CAD build for the part. Positions are in the model's coordinates, mm. A direction names the side the tool comes from. Round coordinates to 2 decimals unless told otherwise and drop trailing zeros. Loops run counter-clockwise (first coordinate to the right, second up) from the corner with the lowest first, then second, coordinate; pieces in that order, holes last. Notation, with made-up numbers: M 2.25,86.5 L 20.25,86.5 A22 ccw 20.25,97.5 Z; hole C 43.25,-13 d6. An arc over 180 degrees is marked long. Put each result on its own line as item: value. Start each with the question number.
Autodesk Inventor part; units mm, degrees
ref_plane "YZ Plane" through (0, 0, 0) normal (1, 0, 0) x (0, 1, 0)
ref_plane "XZ Plane" through (0, 0, 0) normal (0, 1, 0) x (-1, 0, 0)
ref_plane "XY Plane" through (0, 0, 0) normal (0, 0, 1) x (1, 0, 0)
sketch "스케치2" plane through (0, 0, 0) normal (0, 1, 0) x (-1, 0, 0)
  line L0 (0, -70.4) -> (-60.9682, -35.2)
  line L1 (-60.9682, -35.2) -> (-60.9682, 35.2)
  line L2 (-60.9682, 35.2) -> (0, 70.4)
  line L3 (0, 70.4) -> (60.9682, 35.2)
  line L4 (60.9682, 35.2) -> (60.9682, -35.2)
  line L5 (60.9682, -35.2) -> (0, -70.4)
  line L6 (60.9682, -35.2) -> (-60.9682, -35.2)
  line L7 (-60.9682, -35.2) -> (-60.9682, 35.2)
  line L8 (-60.9682, 35.2) -> (60.9682, 35.2)
  line L9 (60.9682, 35.2) -> (60.9682, -35.2)
  line L10 (60.9682, -35.2) -> (-60.9682, 35.2) construction
  line L11 (-60.9682, -35.2) -> (60.9682, 35.2) construction
  line L12 (0, 76.1735) -> (-65.9682, 38.0868)
  line L13 (-65.9682, 38.0868) -> (-65.9682, -38.0868)
  line L14 (-65.9682, -38.0868) -> (0, -76.1735)
  line L15 (0, -76.1735) -> (65.9682, -38.0868)
  line L16 (65.9682, -38.0868) -> (65.9682, 38.0868)
  line L17 (65.9682, 38.0868) -> (0, 76.1735)
  line L18 (49.325, -35.2) -> (-49.325, -35.2)
  line L19 (-49.325, -35.2) -> (-49.325, 35.2)
  line L20 (-49.325, 35.2) -> (49.325, 35.2)
  line L21 (49.325, 35.2) -> (49.325, -35.2)
  line L22 (49.325, -35.2) -> (-49.325, 35.2) construction
  line L23 (-49.325, -35.2) -> (49.325, 35.2) construction
  line L24 (49.325, 35.2) -> (65.9682, 35.2)
  line L25 (65.9682, 35.2) -> (65.9682, 29.2)
  line L26 (65.9682, 29.2) -> (49.325, 29.2)
  line L27 (49.325, 29.2) -> (49.325, 35.2)
  line L28 (49.325, -35.2) -> (65.9682, -35.2)
  line L29 (65.9682, -35.2) -> (65.9682, -29.2)
  line L30 (65.9682, -29.2) -> (49.325, -29.2)
  line L31 (49.325, -29.2) -> (49.325, -35.2)
  line L32 (5.675, -35.2) -> (5.675, -72.897)
  line L33 (-49.325, -25.2) -> (-65.9682, -25.2)
  line L34 (-65.9682, -25.2) -> (-65.9682, -5.2)
  line L35 (-65.9682, -5.2) -> (-49.325, -5.2)
  line L36 (-49.325, -5.2) -> (-49.325, -25.2)
  line L37 (-39.325, -35.2) -> (-39.325, -53.4692)
  point P0 (0, 0)
  point P1 (0, 0)
  dimension "d2" = 70.4
  dimension "d3" = 70.4
  dimension "d4" = 5
  dimension "d5" = 98.65
  dimension "d6" = 6
  dimension "d7" = 6
  dimension "d9" = 10
  dimension "d10" = 30
  dimension "d15" = 10
  dimension "d16" = 55
extrude "돌출1" add sketch "스케치2" along normal blind 32 contours L37 L14 L13 L33 L1 L0 | L0 L6 L37 | L32 L6 L5 | L5 L28 L16 L15 L32 | L1 L33 L19 L6 | L6 L21 L30 L4 | L4 L30 L16 L28 | L35 L13 L12 L17 L16 L24 L3 L2 L1 | L1 L8 L19 L35 | L26 L21 L8 L4 | L4 L24 L16 L26 | L2 L3 L8
sketch "스케치3" plane through (0, 0, 0) normal (0, 1, 0) x (-1, 0, 0)
  line L0 (0, 76.1735) -> (-65.9682, 38.0868) construction
  line L1 (0, 76.1735) -> (65.9682, 38.0868)
  line L2 (65.9682, 38.0868) -> (65.9682, -38.0868)
  line L3 (65.9682, -38.0868) -> (0, -76.1735)
  line L4 (0, -76.1735) -> (-65.9682, -38.0868)
  line L5 (-65.9682, -38.0868) -> (-65.9682, 38.0868)
  line L6 (-65.9682, 38.0868) -> (0, 76.1735)
  point P0 (0, 0)
  point P1 (0, 0)
extrude "돌출2" add sketch "스케치3" against normal blind 5
sketch "스케치4" plane through (0, 32, 0) normal (0, 1, 0) x (1, 0, 0)
  circle A0 centre (0, -55) radius 2.5
  circle A1 centre (-25, 45) radius 2.5
  circle A2 centre (57, 35) radius 2.5
  point P0 (0, 0)
  dimension "d17" = 5
  dimension "d18" = 55
  dimension "d19" = 5
  dimension "d20" = 45
  dimension "d21" = 25
  dimension "d22" = 5
  dimension "d23" = 57
  dimension "d24" = 35
extrude "돌출3" cut sketch "스케치4" against normal blind 5
chamfer "모따기1" distance 1 angle 45 10 edges at (-2.5, 32, 55) (-27.5, 32, -45) (54.5, 32, -35) (-27.5, 32, -35.2) (-49.325, 32, -32.2) (-49.325, 32, 32.2) (0, 32, 35.2) (44.325, 32, -35.2) (49.325, 32, -30.2) (49.325, 32, 15)
equation "\"d3\" = d2"
properties part number "pi_case_bottom"
(1) Cut at B-B on y = 24. List the corners of the cut face in (x, z) (1 decimal), and give its area (3 significant figures).
(2) Cut at D-D on z = -59. List the corners of the cut face in (x, y) (3 decimals).
(3) Cut at C-C on x = -44.5. List the corners of the cut face in (y, z), and give its area (3 significant figures).
(4) Flat gauge pins, fed straight in: pin 1 Ø12 at (x, y) = (33, 13) entering from +Z; pin 2 Ø5.5 at (x, z) = (58, -35.5) entering from +Y; pin 3 Ø9.5 at (x, y) = (-16, 17.5) entering from -Z; pin 4 Ø4 at (x, y) = (-34.5, 26) entering from +Z. Where does each tip first touch, or does it go through?
(5) Cut at A-A on z = 2. List the corners of the cut face in (x, y) (3 decimals).
(6) Drill centre lines: line 1 along X through (y, z) = (29, -35) (3 decimals); line 2 along Z through (x, y) = (0, 29.05); line 3 along Z through (x, y) = (57, 27.85). Where is each one in solid material? Low to high.
(7) Tool access for faces 1 (the flat face through (-32.52, 13.76, 57.4)), 2 (the flat face through (1, 0, -7)), 3 (the flat face through (10, 32, 42)), 4 (the flat face through (58, 16, -5.2)), 5 (the flat face through (-58, 16, 29.2)): list every direction of +Z, -Z, +X, -X, +Y, -Y with a clear straight run to the whole face (end or side of a thin tool).
(8) Mould opens along Z. For faces 6 (the flat face through (49.325, 15, -30)), 7 (the flat face through (39.325, 16, -44)), 8 (the flat face through (-33.45, 13.76, -56.86)) say: +Z half, -Z half, draft (parallel to the pull), parting line (faces both ways), or undercut.
Taken from the geometry:
1. outline: M -66,-38.1 L -5.7,-72.9 L -5.7,-35.2 L -49.3,-35.2 L -49.3,-29.2 L -66,-29.2 Z; M -66,29.2 L -49.3,29.2 L -49.3,35.2 L 49.3,35.2 L 49.3,-5.2 L 66,-5.2 L 66,38.1 L 0,76.2 L -66,38.1 Z; M 39.3,-53.5 L 66,-38.1 L 66,-25.2 L 49.3,-25.2 L 49.3,-35.2 L 39.3,-35.2 Z
1. area: 5,440 mm2
2. outline: M -29.745,-5 L 29.745,-5 L 29.745,0 L -5.675,0 L -5.675,32 L -29.745,32 Z
3. outline: M -5,-50.48 L 32,-50.48 L 32,-36.2 L 31,-35.2 L 0,-35.2 L 0,35.2 L 31,35.2 L 32,36.2 L 32,50.48 L -5,50.48 Z
3. area: 1,480 mm2
4. pin 1: z = 60.59
4. pin 2: y = 32
4. pin 3: z = -69.68
4. pin 4: z = 57.41
5. outline: M -65.968,-5 L 65.968,-5 L 65.968,32 L 50.325,32 L 49.325,31 L 49.325,0 L -65.968,0 Z
6. line 1: -65.968 to -49.325, 49.325 to 54.5, 59.5 to 65.968
6. line 2: 35.2 to 52.5, 57.5 to 76.17
6. line 3: -43.26 to -37.5, -32.5 to -25.2, -5.2 to 43.26
7. face 1: +Z, -X, +Y, -Y
7. face 2: +Y
7. face 3: +Z, -Z, +X, -X, +Y
7. face 4: +X, -X, +Y
7. face 5: -X, +Y
8. face 6: undercut
8. face 7: draft
8. face 8: -Z half
